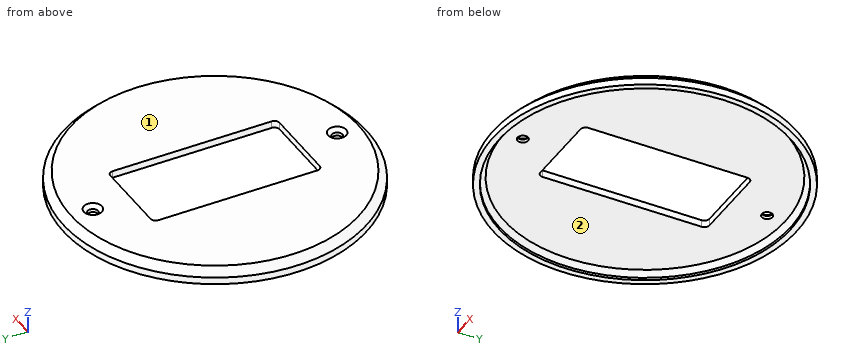
```python
from build123d import *

# Parameters (mm, degrees)
F0_R     = 60
F0_R_2   = 57.6
F0_R_3   = 2.1
F1_DEPTH = 5.8
F2_SIZE  = 3
F3_DEPTH = 3
F4_SIZE  = 2
F5_SIZE  = 1.5


with BuildPart() as f1:
    # F0 (on Top) → F1 (new body)
    with BuildSketch(Plane.XY):
        Circle(F0_R)
        Circle(F0_R_2, mode=Mode.SUBTRACT)
        Circle(F0_R_2)
        with Locations((0, -48.4)):
            Circle(F0_R_3, mode=Mode.SUBTRACT)
        with BuildLine():
            Line((-14.75, 33.5), (14.75, 33.5))
            ThreePointArc((14.75, 33.5), (16.164214, 32.914214), (16.75, 31.5))
            Line((16.75, 31.5), (16.75, -31.5))
            ThreePointArc((16.75, -31.5), (16.164214, -32.914214), (14.75, -33.5))
            Line((14.75, -33.5), (-14.75, -33.5))
            ThreePointArc((-14.75, -33.5), (-16.164214, -32.914214), (-16.75, -31.5))
            Line((-16.75, -31.5), (-16.75, 31.5))
            ThreePointArc((-16.75, 31.5), (-16.164214, 32.914214), (-14.75, 33.5))
        make_face(mode=Mode.SUBTRACT)
        with Locations((0, 48.4)):
            Circle(F0_R_3, mode=Mode.SUBTRACT)
    extrude(amount=F1_DEPTH)

    # F2
    f2_edges = [f1.edges().sort_by_distance(p)[0] for p in [
        (-60, 0, 5.8),
    ]]
    chamfer(f2_edges, length=F2_SIZE)

    # F0 (on Top) → F3 (cut)
    with BuildSketch(Plane.XY):
        Circle(F0_R_2)
        with Locations((0, -48.4)):
            Circle(F0_R_3, mode=Mode.SUBTRACT)
        with BuildLine():
            Line((-14.75, 33.5), (14.75, 33.5))
            ThreePointArc((14.75, 33.5), (16.164214, 32.914214), (16.75, 31.5))
            Line((16.75, 31.5), (16.75, -31.5))
            ThreePointArc((16.75, -31.5), (16.164214, -32.914214), (14.75, -33.5))
            Line((14.75, -33.5), (-14.75, -33.5))
            ThreePointArc((-14.75, -33.5), (-16.164214, -32.914214), (-16.75, -31.5))
            Line((-16.75, -31.5), (-16.75, 31.5))
            ThreePointArc((-16.75, 31.5), (-16.164214, 32.914214), (-14.75, 33.5))
        make_face(mode=Mode.SUBTRACT)
        with Locations((0, 48.4)):
            Circle(F0_R_3, mode=Mode.SUBTRACT)
    extrude(amount=F3_DEPTH, mode=Mode.SUBTRACT)

    # F4
    f4_edges = [f1.edges().sort_by_distance(p)[0] for p in [
        (-57.6, 0, 3),
    ]]
    chamfer(f4_edges, length=F4_SIZE)

    # F5
    f5_edges = [f1.edges().sort_by_distance(p)[0] for p in [
        (-2.1, -48.4, 5.8),
        (-2.1, 48.4, 5.8),
    ]]
    chamfer(f5_edges, length=F5_SIZE)


solid = f1.part
```
The listing builds one solid part. Answer for the finished solid, in the listing's coordinates (mm). Face numbers are marked on the shaded views. Give positions to 0.01 mm unless a question says otherwise; leave off trailing zeros. Order: outer loops, then holes, each group sorted by start corner. A loop starts at its lowest first (then second) coordinate and runs counter-clockwise, first axis right, second up.
1) Find section A-A on y = 0. Write down the section's boundary in (x, z).
Reported:
outline: (-60, 0) - (-57.6, 0) - (-57.6, 1) - (-55.6, 3) - (-16.75, 3) - (-16.75, 5.8) - (-57, 5.8) - (-60, 2.8) - close; (16.75, 3) - (55.6, 3) - (57.6, 1) - (57.6, 0) - (60, 0) - (60, 2.8) - (57, 5.8) - (16.75, 5.8) - close
2) Determine the mould class of the marked faces 1 and 2 for opening direction Y: pulls with the +Y half, pulls with the -Y half, needs draft (parallel to the pull), parting line crosses it, or undercut.
Reported:
face 1: needs draft
face 2: undercut
3) Given P1, Ø3, axis at x = 19, z = 3.5, coming from the +Y side; P2, Ø2, axis at y = -1.5, z = 4.5, coming from the -X side; P3, Ø3, axis at x = 47, y = 26.5, coming from the -Z side, each flat-ended and moving along its own axis, determine where each tip first touches the part or whether it passes through.
Reported:
P1: stops at y = 57.34
P2: stops at x = -59.28
P3: stops at z = 3
4) Consider line 1 along Y through (x, z) = (0, 3.85); line 2 along Y through (x, z) = (0, 3.5); line 3 along Y through (x, z) = (0, 0.25). Determine where each line is inside the solid, lowest interval first.
Reported:
line 1: y = -58.95 to -50.5, -46.3 to -33.5, 33.5 to 46.3, 50.5 to 58.95
line 2: y = -59.3 to -50.5, -46.3 to -33.5, 33.5 to 46.3, 50.5 to 59.3
line 3: y = -60 to -57.6, 57.6 to 60
